Could you check a few things on this drawing? It's one solid part, dimensions in mm from its lowest x, y, z. Round coordinates to 2 decimals unless told otherwise and drop trailing zeros. Loops run counter-clockwise (first coordinate to the right, second up) from the corner with the lowest first, then second, coordinate; pieces in that order, holes last. Notation, with made-up numbers: M 58,12.5 L 64,12.5 A13 ccw 64,23.5 Z; hole C 75.25,-12 d6. An arc over 180 degrees is marked long. Use a Markdown table: item, result. Add a question column.
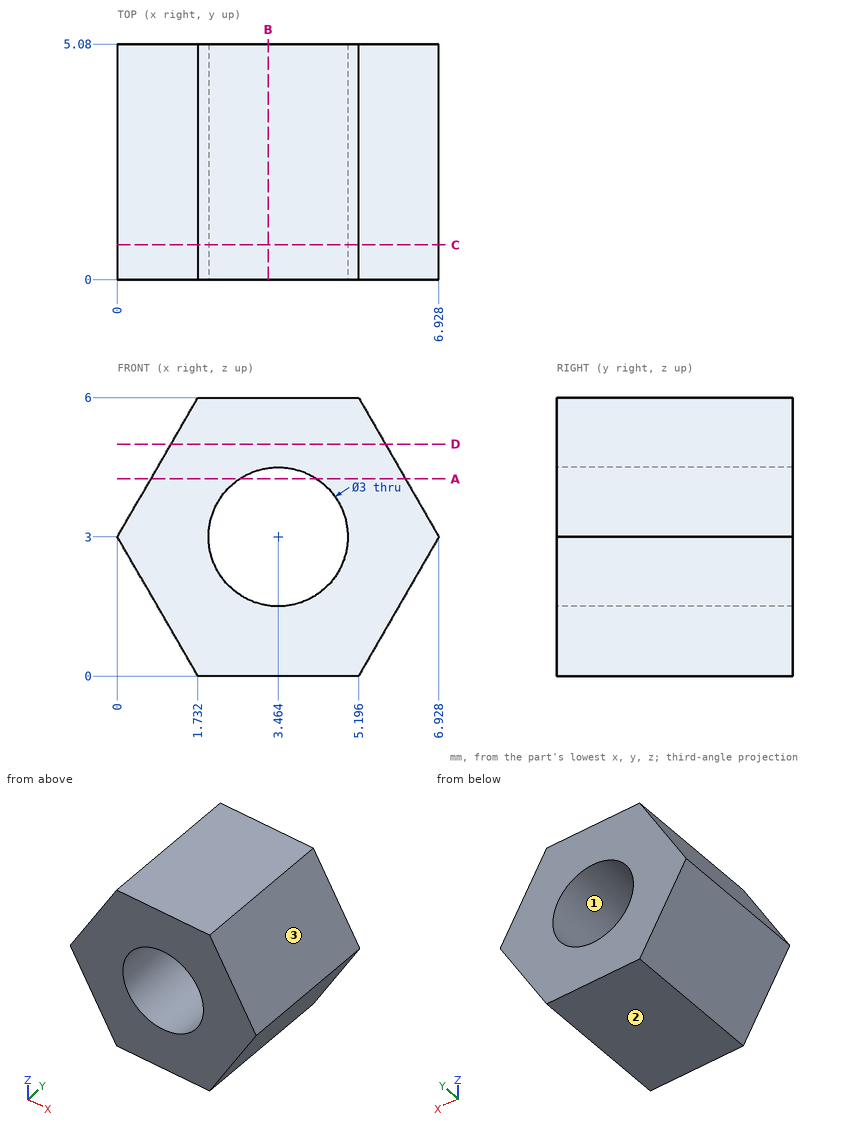
(1) If I drill on probe 1 along X at (y, z) = (3.55, 3.5); probe 2 along Z at (x, y) = (4, 4.6); probe 3 along Z at (x, y) = (5.25, 2.7) (1 decimal), over which ranges is the centre line in solid material (lowest first)? Write a range as [from, to].
(2) Suppose I cut it at A-A on z = 4.25. List the corners of the cut face in (x, y) for me (1 decimal).
(3) Thinking about a two-plate mould opening in X: for the marked faces 1, 2 and 3, which applies, released by +X, released by -X, zero draft, split by the parting line, or undercut?
(4) Suppose I cut it at B-B on x = 3.25. List the corners of the cut face in (y, z) for me (1 decimal).
(5) Suppose I cut it at C-C on y = 0.75. List the corners of the cut face in (x, z) for me.
(6) Suppose I cut it at D-D on z = 5. List the corners of the cut face in (x, y) for me (1 decimal), and give its area (3 significant figures).
Results below:
| question | item | result |
|---|---|---|
| 1 | probe 1 | x = [0.29, 2.05], [4.88, 6.64] |
| 1 | probe 2 | z = [0, 1.6], [4.4, 6] |
| 1 | probe 3 | z = [0.1, 5.9] |
| 2 | outline | M 0.7,0 L 2.6,0 L 2.6,5.1 L 0.7,5.1 Z; M 4.3,0 L 6.2,0 L 6.2,5.1 L 4.3,5.1 Z |
| 3 | face 1 | undercut |
| 3 | face 2 | zero draft |
| 3 | face 3 | released by +X |
| 4 | outline | M 0,0 L 5.1,0 L 5.1,1.5 L 0,1.5 Z; M 0,4.5 L 5.1,4.5 L 5.1,6 L 0,6 Z |
| 5 | outline | M 0,3 L 1.73,0 L 5.2,0 L 6.93,3 L 5.2,6 L 1.73,6 Z; hole C 3.46,3 d3 |
| 6 | outline | M 1.2,0 L 5.8,0 L 5.8,5.1 L 1.2,5.1 Z |
| 6 | area | 23.5 mm² |
